The listing builds one solid part. Answer for the finished solid, in the listing's coordinates (mm). A direction names the side the tool comes from. Round coordinates to 2 decimals unless told otherwise and drop trailing zeros. Write each loop counter-clockwise with the first axis right and the second up, starting at its lowest first coordinate (ties: lowest second). Pieces come first, ordered by that corner, then holes. Notation, with made-up numbers: (59, 83.25) - (108, 83.25) arc R11 cw to (108, 98.25) - close; hole circle Ø8 at (52, 9). An arc over 180 degrees is marked (long way). Answer in a Markdown table with one row per item.
from build123d import *

# Parameters (mm, degrees)
F0_R     = 2.25
F1_DEPTH = 3
F2_DEPTH = 12
F3_DEPTH = 25
F4_DEPTH = 1.9
F5_R     = 1.0323234766
F6_DEPTH = 2


with BuildPart() as f1:
    # F0 (on Front) → F1 (new body)
    with BuildSketch(Plane.XZ):
        Polygon((59.1779698418, 31.194587481), (59.1779698418, 31.9005881237), (59.7388577371, 31.8816154154), (60.3070678192, 32.6076158289), (60.8939676434, 33.1560252645), (60.8939676434, 33.94444243), (60.8939676434, 34.9491785137), (61.3608548692, 35.6423513558), (61.6794760284, 36.3066197257), (61.6794760284, 36.964568034), (61.4824255283, 37.650985105), (61.0625805582, 38.6402383967), (60.3881708198, 39.7264862101), (59.7092475961, 40.8400280338), (58.7607938368, 41.9245535961), (57.6865458859, 42.9608735974), (56.131929641, 44.1080185295), (53.9428997059, 45.2900241974), (51.8717793367, 45.8880749855), (51.1641228177, 46.2767657275), (50.0276083315, 47.254787707), (49.500445814, 47.9175015095), (49.1623850594, 48.6403019596), (48.6890909202, 49.5821496811), (48.0721058512, 50.756745827), (47.4028453988, 51.9204250674), (46.7350661522, 52.8268286536), (46.0711401365, 53.7907023235), (45.4648239409, 54.5656838351), (44.6564314585, 55.4715389559), (43.8822848719, 56.1802155505), (42.8986280226, 56.9550049245), (41.9814228134, 57.3815747084), (41.2078828484, 57.4680692876), (40.7050007603, 57.323706376), (40.2931032973, 56.6803844909), (40.199734935, 55.9481483411), (40.199734935, 53.9804748212), (39.6002588357, 54.273896786), (38.8731125838, 54.6692215131), (37.691644901, 55.1789449292), (36.5735721249, 55.6012317928), (35.1899154237, 55.8898272879), (34.2816298321, 55.6290847487), (33.6731372422, 55.1684227791), (33.4962484397, 54.2325872158), (33.6837781683, 52.5928086281), (34.1659036474, 51.3379723538), (34.7663858487, 49.5873513683), (35.2569758596, 48.3876865141), (35.9067640461, 47.0506118809), (36.5332756434, 45.9664146991), (37.3798895218, 44.924222276), (38.3908508618, 44.0280229397), (39.5714766328, 43.2154907668), (40.3047049111, 42.4076781904), (41.0011964924, 41.6110026044), (40.6037128381, 40.9368513783), (40.0780839274, 40.1968563654), (39.8294614492, 39.436208314), (39.5429389686, 38.0218070561), (39.9435562115, 36.928816962), (39.9435562115, 36.0942029461), (39.6868255292, 35.5139231333), (39.2115087057, 34.9491785137), (38.4849423599, 34.4103130735), (37.4947947552, 33.8397134992), (36.2388370964, 33.8397134992), (34.1682477254, 34.1105470766), (31.5846720936, 34.4943121109), (29.9018896319, 34.7448454842), (25.7982475776, 35.2533147662), (22.9338105357, 35.2533147662), (20.4925913511, 35.2533147662), (18.0653283384, 35.0201785734), (15.8854493902, 34.5568092112), (13.8497609292, 33.7397600595), (12.1293465844, 32.6644815528), (10.4578391027, 31.2680783419), (8.8429108853, 29.5349174183), (7.4372964263, 27.5334818399), (6.0921336762, 25.2153127735), (5.626352988, 22.9853138756), (5.2811054162, 22.9853138756), (4.5523054715, 23.3941563518), (3.3652996425, 23.5582872219), (2.3869021215, 22.8734776027), (1.8580647324, 21.2996615779), (1.2503211514, 18.4274045382), (1.3953504937, 15.7512989625), (1.9034004358, 13.1371476651), (2.4727079067, 11.1539892033), (3.5306752582, 9.5370138477), (4.8935674994, 8.138209791), (6.9346738022, 6.4682455231), (7.7356851464, 6.4682455231), (8.3006708113, 6.139061086), (8.7042880198, 4.7330776356), (9.059931979, 3.7272284641), (10.1391117511, 3.1285394737), (12.4473123728, 2.994476163), (14.4526387363, 3.1366197305), (16.8182124996, 3.1366197305), (18.0060434283, 2.8763879966), (19.3903542013, 2.6614952628), (21.883129127, 2.6614952628), (23.7435637012, 2.6614952628), (26.1859881122, 2.6614952628), (28.06579015, 2.8763879966), (29.066299208, 2.8763879966), (30.1331987714, 3.287266694), (30.1331987714, 3.5115652152), (30.1331987714, 4.0722664313), (30.1331987714, 4.7332313456), (29.8045038484, 5.5102918726), (29.2580751761, 6.1180421129), (30.1753048391, 6.385948213), (31.1070111921, 6.7245609263), (32.1866285138, 7.1757989864), (33.3447322722, 7.8400621162), (34.1773899787, 8.6830629355), (34.5961799391, 8.3883274486), (35.2824532969, 7.6921380472), (36.3022424833, 6.5724259885), (37.0747716212, 5.4643229671), (38.0653628889, 4.2985577244), (38.7650963545, 3.287266694), (39.5393966511, 2.1927098055), (40.5617639739, 1.4101439923), (41.8474854837, 1.29517555), (43.3533756495, 1.6162313684), (44.9111674038, 1.6162313684), (45.7386897979, 1.4101439923), (47.1447348197, 1.4101439923), (48.0390547016, 1.8218246455), (48.391113549, 2.4300583955), (48.391113549, 3.1064440938), (49.9711618169, 3.1064440938), (50.7690600963, 3.3749897061), (51.1641228177, 3.7687113949), (51.1641228177, 4.5507251402), (50.8511063176, 5.8227389469), (50.331727117, 6.6105731496), (49.7232345272, 7.1669628431), (48.7272878623, 7.3274251963), (47.8059953638, 7.5314743863), (47.4058916521, 7.9913136579), (47.3091591362, 8.5442592861), (47.0176340929, 9.8221136372), (46.7949781293, 11.4877626708), (46.7949781293, 12.8848767905), (46.9349625513, 13.7100262861), (47.2396647362, 14.3331588828), (48.0156837904, 15.3890061712), (49.3168950791, 17.0124460815), (50.682930079, 19.1019749735), (51.1880177404, 21.1130785633), (51.5269728079, 22.9853138756), (51.9142522124, 24.7934957735), (52.5664263977, 26.5176664071), (53.3611806084, 27.9593477017), (56.4587800437, 29.8548648433), (58.2113468584, 30.3689550216), align=None)
        with Locations((52.3673893774, 39.17497812)):
            Circle(F0_R, mode=Mode.SUBTRACT)
    extrude(amount=F1_DEPTH)

    # F2 (add): a face of the model
    f2_faces = [f1.faces().sort_by_distance(p)[0] for p in [
        (31.8904414267, -3, 24.0565595855),
    ]]
    extrude(f2_faces, amount=F2_DEPTH)

    # F3 (cut): a face of the model
    f3_faces = [f1.faces().sort_by_distance(p)[0] for p in [
        (23.1454194643, -7.5, 35.2533147662),
    ]]
    extrude(f3_faces, amount=-F3_DEPTH, mode=Mode.SUBTRACT)

    # F4 (add): a face of the model
    f4_faces = [f1.faces().sort_by_distance(p)[0] for p in [
        (20.4925913511, -7.5, 22.7533147662),
    ]]
    extrude(f4_faces, amount=F4_DEPTH)

    # F5 (on face) → F6 (join)
    with BuildSketch(Plane.XZ.offset(15)):
        with Locations((41.8074317276, 54.3998554349)):
            Circle(F5_R)
    extrude(amount=-F6_DEPTH)


solid = f1.part
(1) For faces 4 (the flat face through (23, -7, 2.661)), 5 (the flat face through (21, -7, 35.253)), 6 (the flat face through (33.59, -7.4, 53.42)), 7 (the flat face through (50.93, -7.4, 20.09)), 8 (the flat face through (30.133, -7, 4)), determine the directions among +Z, -Z, +X, -X, +Y, -Y from which every point of the face is accessible in a straight line to the end or side of a thin tool.
Checked values:
| item | result |
|---|---|
| face 4 | -Z, -X, +Y, -Y |
| face 5 | +Z, -X, +Y, -Y |
| face 6 | -X, +Y, -Y |
| face 7 | +X, +Y, -Y |
| face 8 | -Z, +Y, -Y |
(2) Flat-ended cylindrical pins translate along their axes: pin 1 (10 mm diameter, centred on x = 22.5, z = 20, fed in from -Y); pin 2 (1.7 mm diameter, centred on x = 24.5, y = -7, fed in from +Z); pin 3 (0.6 mm diameter, centred on y = -4, z = 31.5, fed in from +X); pin 4 (1.4 mm diameter, centred on y = -7, z = 34.5, fed in from +X). Find the tip coordinate at first contact, or state that the pin passes through.
Checked values:
| item | result |
|---|---|
| pin 1 | stops at y = -15 |
| pin 2 | stops at z = 10.25 |
| pin 3 | stops at x = 59.18 |
| pin 4 | stops at x = 61.06 |
(3) For a pull along Z with two mould halves and no side action, classify faces 1 (the flat face through (5.863, -7.395, 24.116)), 2 (the flat face through (31, 0, 24)), 3 (the flat face through (51.01, -7.4, 5.18)) as pulls with the +Z half, pulls with the -Z half, needs draft (parallel to the pull), parting line crosses it, or undercut.
Checked values:
| item | result |
|---|---|
| face 1 | pulls with the +Z half |
| face 2 | needs draft |
| face 3 | undercut |
(4) Find the intervals of material crossed by line 1 (Z direction, x = 21, y = -7.5); line 2 (X direction, y = -5, z = 4.5); line 3 (X direction, y = -3.25, z = 22.5), in increasing order.
Checked values:
| item | result |
|---|---|
| line 1 | z = 2.66 to 35.25 |
| line 2 | x = 8.79 to 30.13, 37.89 to 51.16 |
| line 3 | x = 2.26 to 22.39, 25.8 to 51.44 |
(5) Section A-A (x = 27) is taken. Give the vertices of the cut face in (y, z).
Checked values:
| item | result |
|---|---|
| outline | (-15, 2.75) - (0, 2.75) - (0, 35.1) - (-15, 35.1) - close |
